from build123d import *

# Parameters (mm, degrees)
F0_R     = 254
F1_DEPTH = 1524
F3_DEPTH = 381


with BuildPart() as f1:
    # F0 (on Front) → F1 (new body)
    with BuildSketch(Plane.XZ):
        Circle(F0_R)
    extrude(amount=F1_DEPTH)

    # F2 (on face) → F3 (join)
    with BuildSketch(Plane.XZ.offset(1524)):
        Polygon((241.568355, 78.490317), (0, 254), (-241.568355, 78.490317), (-149.297454, -205.490317), (149.297454, -205.490317), align=None)
    extrude(amount=F3_DEPTH)


solid = f1.part
Here's how the part is built. I have some questions about the finished solid (model axes, mm). A direction names the side the tool comes from. Give positions to 0.01 mm unless a question says otherwise; leave off trailing zeros. Order: outer loops, then holes, each group sorted by start corner. A loop starts at its lowest first (then second) coordinate and runs counter-clockwise, first axis right, second up. Notation, with made-up numbers: M -23.5,32 L 16.5,32 A15 ccw 16.5,53 Z; hole C 26,-19.75 d8. An arc over 180 degrees is marked long. Answer as a JSON object with one key per item and string values. Group by question number.
1) Suppose I cut it at B-B, the plane x = 62.5. Write out the boundary of the cut face in (y, z).
2) Please list where these lines run through material, in increasing order: L1, parallel to Z at x = 11, y = -726.5; L2, parallel to Y at x = 89, z = -212.5; L3, parallel to X at y = -567, z = 208.5. Write a range as [from, to].
3) Suppose I cut it at A-A, the plane z = -102. Write out the boundary of the cut face in (x, y), plus the area to 3 significant figures.
4) On a 3-axis mill with a long thin cutter (end or side, diameter ignored), from which of +Z, -Z, +X, -X, +Y, -Y can I reach the whole of each face in a straight line? I mean faces 1 (the flat face through (-2, -1712, -205.49)), 2 (the flat face through (129, -1524, 180)), 3 (the flat face through (-196.08, -1711.83, -61.51)), 4 (the flat face through (194.787, -1711.833, -65.488)). Say none if no direction works.
5) Suppose I cut it at C-C, the plane y = -290. Write out the boundary of the cut face in (x, z), plus the area to 3 significant figures.
6) I'm going to push flat-ended pins straight in: pin 1 Ø1 at (x, y) = (-176.5, -1172.5) entering from -Z; pin 2 Ø1 at (x, y) = (76, -1704.5) entering from +Z; pin 3 Ø2 at (y, z) = (-869, -147) entering from +X. Where does each tip first touch, or does it pass through?
Results found:
{
 "1": {"outline": "M -1905,-205.49 L -1524,-205.49 L -1524,-246.19 L 0,-246.19 L 0,246.19 L -1524,246.19 L -1524,208.59 L -1905,208.59 Z"},
 "2": {"L1": "[-253.76, 253.76]", "L2": "[-1524, 0]", "L3": "[-145.06, 145.06]"},
 "3": {"outline": "M -232.62,-1524 L -182.92,-1524 L -182.92,-1905 L 182.92,-1905 L 182.92,-1524 L 232.62,-1524 L 232.62,0 L -232.62,0 Z", "area": "848,000 mm²"},
 "4": {"face 1": "-Z, +X, -X, -Y", "face 2": "+Z, +X, -Y", "face 3": "-Z, -X, -Y", "face 4": "-Z, +X, -Y"},
 "5": {"outline": "C 0,0 d508", "area": "203,000 mm²"},
 "6": {"pin 1": "z = -183.14", "pin 2": "z = 199.15", "pin 3": "x = 207.85"}
}
